Here's how the part is built. I have some questions about the finished solid (model axes, mm). A direction names the side the tool comes from. Coordinates: 2 decimals unless noted, no trailing zeros. Write each loop counter-clockwise with the first axis right and the second up, starting at its lowest first coordinate (ties: lowest second). Pieces come first, ordered by that corner, then holes. Notation, with made-up numbers: M -1.75,85.25 L 13.25,85.25 A21 ccw 13.25,124.25 Z; hole C 65,27.5 d8. An arc over 180 degrees is marked long. Use a Markdown table: item, result.
```python
from build123d import *

# Parameters (mm, degrees)
SKETCH2_R           = 2.275
SKETCH2_W           = 75.079254151
SKETCH2_H           = 30.3
BOSS_EXTRUDE1_DEPTH = 4
SKETCH3_W           = 86
SKETCH3_H           = 4
BOSS_EXTRUDE2_DEPTH = 10


with BuildPart() as part:
    # Sketch2 → Boss-Extrude1 (new body)
    with BuildSketch(Plane(origin=(0, 0, 0), x_dir=(1, 0, 0), z_dir=(0, 1, 0))):
        Polygon((43, 30), (39, 30), (39, 23.15), (-39, 23.15), (-39, 30), (-43, 30), (-43, -30), (-38, -30), (-38, -23.15), (38, -23.15), (38, -30), (43, -30), align=None)
        with Locations(Location((-25.775, 19.15, 0), (0, 0, 270))):
            Circle(SKETCH2_R, mode=Mode.SUBTRACT)
        with Locations(Location((22.854254151, 19.15, 0), (0, 0, 270))):
            Circle(SKETCH2_R, mode=Mode.SUBTRACT)
        with Locations(Location((0, 19.15, 0), (0, 0, 270))):
            Circle(SKETCH2_R, mode=Mode.SUBTRACT)
        with Locations(Location((22.854254151, -19.15, 0), (0, 0, 90))):
            Circle(SKETCH2_R, mode=Mode.SUBTRACT)
        with Locations(Location((0, -19.15, 0), (0, 0, 90))):
            Circle(SKETCH2_R, mode=Mode.SUBTRACT)
        with Locations(Location((-25.775, -19.15, 0), (0, 0, 90))):
            Circle(SKETCH2_R, mode=Mode.SUBTRACT)
        with Locations((-1.460372924, 0)):
            Rectangle(SKETCH2_W, SKETCH2_H, mode=Mode.SUBTRACT)
    extrude(amount=BOSS_EXTRUDE1_DEPTH)

    # Sketch3 → Boss-Extrude2 (add)
    with BuildSketch(Plane(origin=(0, 0, -30), x_dir=(-1, 0, 0), z_dir=(0, 0, -1))):
        with Locations((0, 2)):
            Rectangle(SKETCH3_W, SKETCH3_H)
    extrude(amount=BOSS_EXTRUDE2_DEPTH)


solid = part.part
```
1. Which directions (+Z, -Z, +X, -X, +Y, -Y) give clear straight access to the entire face, cutting with the end or side of a thin tool? Please do faces 4 (the face through (-39, 2, 0)), 5 (the face through (-1, 2, 23.15)), 6 (the face through (10, 0, -20)).
Answers follow:
| item | result |
|---|---|
| face 4 | +Y, -Y |
| face 5 | +Z, +Y, -Y |
| face 6 | +Z, -Z, +X, -X, -Y |
2. Will this pin go through, and if not, where does the flat tip stop? pin 1 Ø5 at (x, z) = (22.85, -19.15) entering from +Y.
Answers follow:
| item | result |
|---|---|
| pin 1 | stops at y = 4 |
3. Suppose I cut it at C-C on z = 19.15. Write out the boundary of the cut face in (x, y) (3 decimals), and give its area (3 significant figures).
Answers follow:
| item | result |
|---|---|
| outline | M -43,0 L -28.05,0 L -28.05,4 L -43,4 Z; M -23.5,0 L -2.275,0 L -2.275,4 L -23.5,4 Z; M 2.275,0 L 20.579,0 L 20.579,4 L 2.275,4 Z; M 25.129,0 L 43,0 L 43,4 L 25.129,4 Z |
| area | 289 mm2 |
4. Suppose I cut it at B-B on x = 0. Write out the boundary of the cut face in (y, z) (3 decimals).
Answers follow:
| item | result |
|---|---|
| outline | M 0,-40 L 4,-40 L 4,-30 L 0,-30 Z; M 0,-23.15 L 4,-23.15 L 4,-21.425 L 0,-21.425 Z; M 0,-16.875 L 4,-16.875 L 4,-15.15 L 0,-15.15 Z; M 0,15.15 L 4,15.15 L 4,16.875 L 0,16.875 Z; M 0,21.425 L 4,21.425 L 4,23.15 L 0,23.15 Z |
5. We'd pull the mould along Z, two halves only. Please class faces 1 (the face through (40, 2, 30)), 2 (the face through (-2, 2, -15.15)), 3 (the face through (38, 2, 27)): +Z half, -Z half, draft (parallel to the pull), parting line (faces both ways), or undercut.
Answers follow:
| item | result |
|---|---|
| face 1 | +Z half |
| face 2 | undercut |
| face 3 | draft |
6. Suppose I cut it at A-A on z = 0. Write out the boundary of the cut face in (x, y), and give its area (3 significant figures).
Answers follow:
| item | result |
|---|---|
| outline | M -43,0 L -39,0 L -39,4 L -43,4 Z; M 36.08,0 L 43,0 L 43,4 L 36.08,4 Z |
| area | 43.7 mm2 |
7. Suppose I cut it at D-D on y = 1.55. State how many separate pieces and enclosed holes the cut face has, and give its area (3 significant figures).
Answers follow:
| item | result |
|---|---|
| separate pieces | 1 |
| enclosed holes | 8 |
| area | 2,590 mm2 |
8. I need wall thicknesses on probe 1 along Z at (x, y) = (-25.5, 1.35); probe 2 along Z at (x, y) = (14, 2.1); probe 3 along X at (y, z) = (2.6, -19.15) (3 decimals). Which ranges of each line are inside material? Lowest first, please.
Answers follow:
| item | result |
|---|---|
| probe 1 | z = -40 to -30, -23.15 to -21.41, -16.89 to -15.15, 15.15 to 16.89, 21.41 to 23.15 |
| probe 2 | z = -40 to -30, -23.15 to -15.15, 15.15 to 23.15 |
| probe 3 | x = -43 to -28.05, -23.5 to -2.275, 2.275 to 20.579, 25.129 to 43 |
